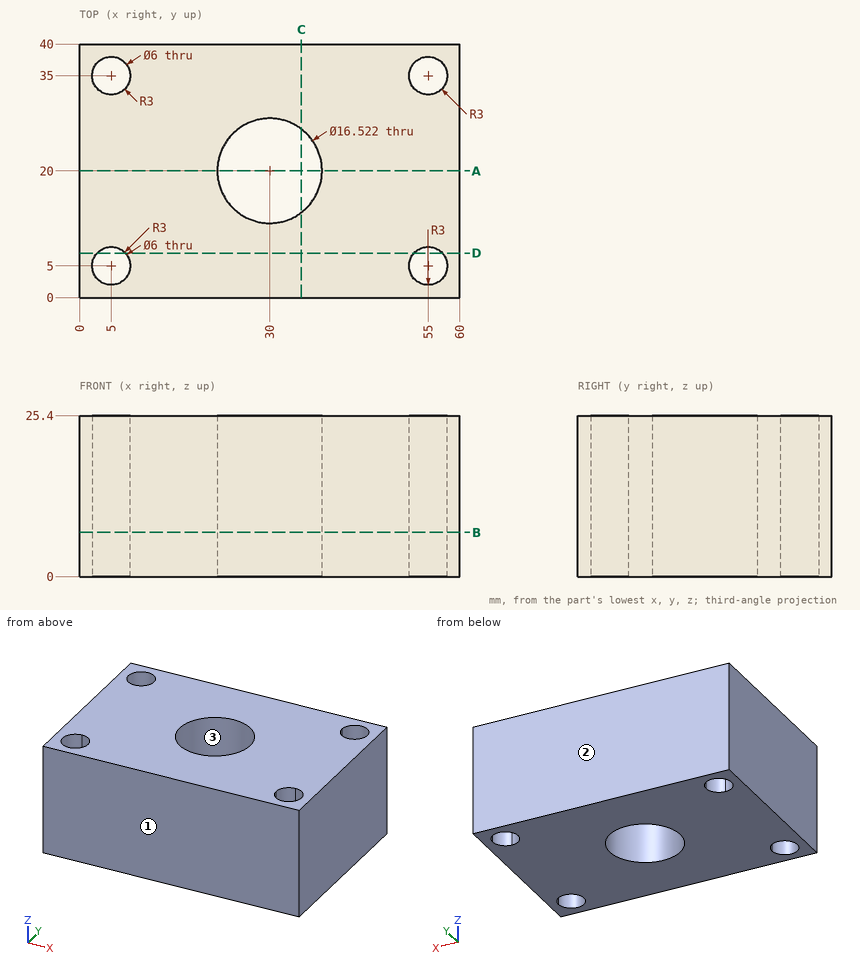
Input: dimensioned drawing with shaded views. Units: mm. Origin: part minimum x, y, z. Round coordinates to 2 decimals unless told otherwise and drop trailing zeros. Loops run counter-clockwise (first coordinate to the right, second up) from the corner with the lowest first, then second, coordinate; pieces in that order, holes last. Notation, with made-up numbers: (-21, -28.5) -> (21, -28.5) arc R29 cw to (21, -8.5) -> close; hole circle Ø6 at (58, 57.5). An arc over 180 degrees is marked (long way). Answer as a JSON object with one key per item and string values. Group by question number.
Q1. Section query C-C (x = 35). Output: boundary loops of the cut face in (y, z).
Q2. Ray query, line 1 (Y direction, x = 5, z = 17.75); line 2 (X direction, y = 5, z = 20.25); line 3 (X direction, y = 7, z = 9). Return the intervals inside material, ascending. Write a range as from..to.
Q3. Section query A-A (y = 20). Output: boundary loops of the cut face in (x, z).
Q4. Mould query, pull axis Y, two halves, no side actions, for the marked faces 1, 2 and 3. Classes: pulls with the +Y half, pulls with the -Y half, needs draft (parallel to the pull), parting line crosses it, or undercut.
Q5. Section query D-D (y = 7). Output: boundary loops of the cut face in (x, z).
Q6. Section query B-B (z = 7). Output: boundary loops of the cut face in (x, y), plus the area to 3 significant figures.
Completed:
{
 "1": {"outline": "(0, 0) -> (13.42, 0) -> (13.42, 25.4) -> (0, 25.4) -> close; (26.58, 0) -> (40, 0) -> (40, 25.4) -> (26.58, 25.4) -> close"},
 "2": {"line 1": "0..2, 8..32, 38..40", "line 2": "0..2, 8..52, 58..60", "line 3": "0..2.76, 7.24..52.76, 57.24..60"},
 "3": {"outline": "(0, 0) -> (21.74, 0) -> (21.74, 25.4) -> (0, 25.4) -> close; (38.26, 0) -> (60, 0) -> (60, 25.4) -> (38.26, 25.4) -> close"},
 "4": {"face 1": "pulls with the -Y half", "face 2": "pulls with the +Y half", "face 3": "undercut"},
 "5": {"outline": "(0, 0) -> (2.76, 0) -> (2.76, 25.4) -> (0, 25.4) -> close; (7.24, 0) -> (52.76, 0) -> (52.76, 25.4) -> (7.24, 25.4) -> close; (57.24, 0) -> (60, 0) -> (60, 25.4) -> (57.24, 25.4) -> close"},
 "6": {"outline": "(0, 0) -> (60, 0) -> (60, 40) -> (0, 40) -> close; hole (5, 8) arc R3 ccw (long way) to (8, 5) arc R3 ccw to start; hole (5, 32) arc R3 ccw to (8, 35) arc R3 ccw (long way) to start; hole circle Ø16.52 at (30, 20); hole (52, 5) arc R3 ccw to (58, 5) arc R3 ccw to (55, 8) arc R3 ccw to start; hole (52, 35) arc R3 ccw to (55, 32) arc R3 ccw to (58, 35) arc R3 ccw to start", "area": "2,070 mm²"}
}
